Geometry check sheet. Reference: the model listing, model coordinates, mm. Face numbers are marked on the shaded views. A direction names the side the tool comes from. Round coordinates to 2 decimals unless told otherwise and drop trailing zeros. Write each loop counter-clockwise with the first axis right and the second up, starting at its lowest first coordinate (ties: lowest second). Pieces come first, ordered by that corner, then holes.
Item 1: Scan lines: probe 1 along Z at (x, y) = (7.5, 4.1); probe 2 along Y at (x, z) = (-2.5, 1.2); probe 3 along Z at (x, y) = (-3.5, 11.6). Record each from-to range of solid material in increasing order.
Item 2: Cross-section at A-A (x = 7.5). Enter the section's corners in (y, z).
Item 3: Access from +Z, -Z, +X, -X, +Y, -Y to the whole of each face (thin tool, end or side, straight path). Record for the marked faces 5, 6, 7 and 8.
Item 4: Cross-section at D-D (x = -3.5). Enter the section's corners in (y, z).
Item 5: Depth check by flat-ended pin: P1, Ø3.5, axis at x = 7, y = 1, coming from the +Z side; P2, Ø1, axis at x = -1.5, y = 1, coming from the -Z side; P3, Ø3, axis at y = -3.5, z = -2, coming from the -X side. Enter the tip coordinate at first touch or a pass-through.
Item 6: Cross-section at C-C (y = 5.25). Enter the section's corners in (x, z), then the cut area to 3 significant figures.
Item 7: Draft check along Z on the marked faces 1, 2, 3 and 4. Enter one of: pulls with the +Z half, pulls with the -Z half, needs draft (parallel to the pull), parting line crosses it, or undercut.
Item 8: Cross-section at B-B (z = 1). Enter the section's corners in (x, y).
from build123d import *

# Parameters (mm, degrees)
ESBO_O1_R                = 1.65
RESSALTO_EXTRUS_O1_DEPTH = 3
ESBO_O3_R                = 1.65
RESSALTO_EXTRUS_O2_DEPTH = 14
ESBO_O4_W                = 5.5
ESBO_O4_H                = 4.2
CORTE_EXTRUS_O1_DEPTH    = 10
ESBO_O5_R                = 1.7
RESSALTO_EXTRUS_O3_DEPTH = 3


with BuildPart() as part:
    # Esboço1 → Ressalto-extrusão1 (new body)
    with BuildSketch(Plane.XY):
        with BuildLine():
            Line((-2.5, -7), (2.5, -7))
            Line((2.5, -7), (12.5, -7))
            Line((12.5, -7), (12.5, 13))
            Line((12.5, 13), (-9.5, 13))
            Line((-9.5, 13), (-9.5, 0))
            ThreePointArc((-9.5, 0), (-7.449747468, -4.949747468), (-2.5, -7))
        make_face()
        with Locations((-2.5, 0)):
            Circle(ESBO_O1_R, mode=Mode.SUBTRACT)
    extrude(amount=RESSALTO_EXTRUS_O1_DEPTH)

    # Esboço3 → Ressalto-extrusão2 (add)
    with BuildSketch(Plane(origin=(0, -7, 0), x_dir=(1, 0, 0), z_dir=(0, 1, 0))):
        with BuildLine():
            Line((2.5, 4), (2.5, 0))
            Line((2.5, 0), (12.5, 0))
            Line((12.5, 0), (12.5, 4))
            ThreePointArc((12.5, 4), (7.5, 9), (2.5, 4))
        make_face()
        with Locations((7.5, 4)):
            Circle(ESBO_O3_R, mode=Mode.SUBTRACT)
    extrude(amount=RESSALTO_EXTRUS_O2_DEPTH)

    # Esboço4 → Corte-extrusão1 (cut)
    with BuildSketch(Plane(origin=(12.5, 0, 0), x_dir=(0, 0, -1), z_dir=(1, 0, 0))):
        with Locations((4, 0)):
            Rectangle(ESBO_O4_W, ESBO_O4_H)
    extrude(amount=-CORTE_EXTRUS_O1_DEPTH, mode=Mode.SUBTRACT)

    # Esboço5 → Ressalto-extrusão3 (add)
    with BuildSketch(Plane(origin=(0, 13, 0), x_dir=(1, 0, 0), z_dir=(0, 1, 0))):
        with BuildLine():
            Line((2.5, 0), (2.5, -13))
            ThreePointArc((2.5, -13), (-3.5, -19), (-9.5, -13))
            Line((-9.5, -13), (-9.5, 0))
            Line((-9.5, 0), (2.5, 0))
        make_face()
        with Locations((-3.5, -13)):
            Circle(ESBO_O5_R, mode=Mode.SUBTRACT)
    extrude(amount=-RESSALTO_EXTRUS_O3_DEPTH)


solid = part.part
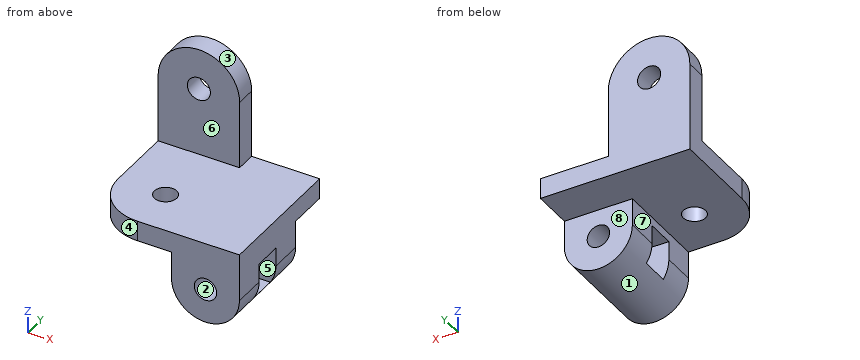
Resolved:
1. probe 1: z = -9 to -5.65, -2.35 to 3
1. probe 2: y = -7 to -1.65, 1.65 to 13
1. probe 3: z = 0 to 11.3, 14.7 to 19
2. outline: (-7, -9) - (7, -9) - (7, -5.65) - (2.1, -5.65) - (2.1, -6.75) - (-2.1, -6.75) - (-2.1, -5.65) - (-7, -5.65) - close; (-7, -2.35) - (-2.1, -2.35) - (-2.1, -1.25) - (2.1, -1.25) - (2.1, -2.35) - (7, -2.35) - (7, 0) - (13, 0) - (13, 3) - (-7, 3) - close
3. face 5: +X, -X
3. face 6: +Z, +X, -X, -Y
3. face 7: -Z, -X, +Y, -Y
3. face 8: -Z, +X, -X, +Y
4. outline: (-6.93, 0) - (-1.31, 0) - (-1.31, 3) - (-6.93, 3) - close; (1.31, 0) - (13, 0) - (13, 11.3) - (10, 11.3) - (10, 3) - (1.31, 3) - close; (10, 14.7) - (13, 14.7) - (13, 19) - (10, 19) - close
5. P1: stops at z = 3
5. P2: stops at z = 0
5. P3: stops at x = 2.5
6. outline: (-9.5, 0) - (2.5, 0) - (2.5, -4) arc R5 ccw to (12.5, -4) - (12.5, 3) - (-9.5, 3) - close; hole circle Ø3.3 at (7.5, -4)
6. area: 137 mm2
7. face 1: pulls with the -Z half
7. face 2: undercut
7. face 3: pulls with the +Z half
7. face 4: needs draft
8. outline: (-9.5, 0) arc R7 ccw to (-2.5, -7) - (12.5, -7) - (12.5, 13) - (-9.5, 13) - close; hole circle Ø3.3 at (-2.5, 0)
